Check sheet for the modelled part. Datum: model origin and axes. Units: mm. A direction names the side the tool comes from. Round coordinates to 2 decimals unless told otherwise and drop trailing zeros. Loops run counter-clockwise (first coordinate to the right, second up) from the corner with the lowest first, then second, coordinate; pieces in that order, holes last. Notation, with made-up numbers: (63.5, -22.75) -> (121.5, -22.75) arc R29 cw to (121.5, 9.25) -> close; hole circle Ø11 at (-22, -3). An arc over 180 degrees is marked (long way). Return JSON: item names as keys, results as strings.
from build123d import *

# Parameters (mm, degrees)
F0_R     = 50
F1_DEPTH = 6
F2_R     = 3
F3_DEPTH = 6
F5_DEPTH = 6


with BuildPart() as f1:
    # F0 (on Top) → F1 (new body)
    with BuildSketch(Plane.XY):
        Circle(F0_R)
    extrude(amount=F1_DEPTH)

    # F2 (on face) → F3 (cut, through all)
    with BuildSketch(Plane(origin=(0, 0, 0), x_dir=(1, 0, 0), z_dir=(0, 0, -1))):
        Circle(F2_R)
    extrude(amount=-F3_DEPTH, mode=Mode.SUBTRACT)

    # F4 (on face) → F5 (cut, through all)
    with BuildSketch(Plane(origin=(0, 0, 0), x_dir=(1, 0, 0), z_dir=(0, 0, -1))):
        with BuildLine():
            Line((-1, 45.989129), (1, 45.989129))
            Line((1, 45.989129), (2.438188, 49.940517))
            ThreePointArc((2.438188, 49.940517), (0, 50.729887), (-2.438188, 49.940517))
            Line((-2.438188, 49.940517), (-1, 45.989129))
        make_face()
    extrude(amount=-F5_DEPTH, mode=Mode.SUBTRACT)


solid = f1.part
Q1. Go/stop test with flat-tipped pins: pin 1 (1.5 mm diameter, centred on x = -8.5, z = 1, fed in from +Y); pin 2 (2 mm diameter, centred on y = -19, z = 5, fed in from -X); pin 3 (1.6 mm diameter, centred on x = 0, z = 2.5, fed in from -Y). Record where each tip stops, or that it passes through.
Results list:
{"pin 1": "y = 49.4", "pin 2": "x = -46.65", "pin 3": "y = -45.99"}
Q2. Draft check along X on faces 1 (the flat face through (-1, -10, 6)), 2 (the flat face through (-1.73, -47.99, 2.96)). Enter one of: released by +X, released by -X, zero draft, split by the parting line, or undercut.
Results list:
{"face 1": "zero draft", "face 2": "undercut"}
Q3. Tool access check on faces 3 (the cylindrical face through (-3, 0, 3)), 4 (the flat face through (1.71, -47.94, 2.96)). Record the directions out of +Z, -Z, +X, -X, +Y, -Y that give a thin tool (end or side, any length) a straight path to the whole face; none if there is none.
Results list:
{"face 3": "+Z, -Z", "face 4": "+Z, -Z, -Y"}
Q4. Material ranges on line 1 (X direction, y = 0, z = 1.9); line 2 (Y direction, x = 0, z = 2.2); line 3 (Y direction, x = -31, z = 4.75), recorded low to high.
Results list:
{"line 1": "-50 to -3, 3 to 50", "line 2": "-45.99 to -3, 3 to 50", "line 3": "-39.23 to 39.23"}
Q5. Section check C-C (x = 23.5). Record the boundary of the cut face in (y, z).
Results list:
{"outline": "(-44.13, 0) -> (44.13, 0) -> (44.13, 6) -> (-44.13, 6) -> close"}
Q6. Section check B-B (y = 27). Record the boundary of the cut face in (x, z).
Results list:
{"outline": "(-42.08, 0) -> (42.08, 0) -> (42.08, 6) -> (-42.08, 6) -> close"}
Q7. Section check A-A (z = 1.2). Record the boundary of the cut face in (x, y), then the cut area to 3 significant figures.
Results list:
{"outline": "(-2.44, -49.94) -> (-1, -45.99) -> (1, -45.99) -> (2.44, -49.94) arc R50 ccw (long way) to start; hole circle Ø6 at (0, 0)", "area": "7,810 mm^2"}
